```python
from build123d import *

# Parameters (mm, degrees)
CROQUIS1_W              = 30
CROQUIS1_H              = 35
CROQUIS1_R              = 1.5
CROQUIS1_R_2            = 2
SALIENTE_EXTRUIR1_DEPTH = 20
CROQUIS2_W              = 10
CROQUIS2_H              = 4
CORTAR_EXTRUIR1_DEPTH   = 41
CORTAR_EXTRUIR2_DEPTH   = 2
CORTAR_EXTRUIR3_DEPTH   = 3
CORTAR_EXTRUIR4_DEPTH   = 3
REDONDEO1_R             = 5
CROQUIS6_W              = 30
CROQUIS6_H              = 11
SALIENTE_EXTRUIR2_DEPTH = 10


with BuildPart() as part:
    # Croquis1 → Saliente-Extruir1 (new body)
    with BuildSketch(Plane(origin=(0, 0, 0), x_dir=(1, 0, 0), z_dir=(0, 1, 0))):
        with Locations((15, 17.5)):
            Rectangle(CROQUIS1_W, CROQUIS1_H)
        with Locations(Location((25, 30, 0), (0, 0, 270))):
            Circle(CROQUIS1_R, mode=Mode.SUBTRACT)
        with Locations(Location((5, 30, 0), (0, 0, 270))):
            Circle(CROQUIS1_R, mode=Mode.SUBTRACT)
        with Locations(Location((7.5, 5, 0), (0, 0, 270))):
            Circle(CROQUIS1_R_2, mode=Mode.SUBTRACT)
        with Locations(Location((22.5, 5, 0), (0, 0, 270))):
            Circle(CROQUIS1_R_2, mode=Mode.SUBTRACT)
    extrude(amount=SALIENTE_EXTRUIR1_DEPTH)

    # Croquis2 → Cortar-Extruir1 (cut)
    with BuildSketch(Plane(origin=(30, 0, 0), x_dir=(0, 0, -1), z_dir=(1, 0, 0))):
        with Locations((30, 13)):
            Rectangle(CROQUIS2_W, CROQUIS2_H)
    extrude(amount=-CORTAR_EXTRUIR1_DEPTH, mode=Mode.SUBTRACT)

    # Croquis3 → Cortar-Extruir2 (cut)
    with BuildSketch(Plane.XZ):
        Polygon((5, -33.117691454), (7.7, -31.558845727), (7.7, -28.441154273), (5, -26.882308546), (2.3, -28.441154273), (2.3, -31.558845727), align=None)
        Polygon((25, -33.117691454), (27.7, -31.558845727), (27.7, -28.441154273), (25, -26.882308546), (22.3, -28.441154273), (22.3, -31.558845727), align=None)
    extrude(amount=-CORTAR_EXTRUIR2_DEPTH, mode=Mode.SUBTRACT)

    # Croquis4 → Cortar-Extruir3 (cut)
    with BuildSketch(Plane.XZ):
        Polygon((7.5, -8.983716857), (10.95, -6.991858429), (10.95, -3.008141571), (7.5, -1.016283143), (4.05, -3.008141571), (4.05, -6.991858429), align=None)
        Polygon((22.5, -8.983716857), (25.95, -6.991858429), (25.95, -3.008141571), (22.5, -1.016283143), (19.05, -3.008141571), (19.05, -6.991858429), align=None)
    extrude(amount=-CORTAR_EXTRUIR3_DEPTH, mode=Mode.SUBTRACT)

    # Croquis5 → Cortar-Extruir4 (cut)
    with BuildSketch(Plane(origin=(0, 20, 0), x_dir=(1, 0, 0), z_dir=(0, 1, 0))):
        Polygon((22.5, 1.016283143), (19.05, 3.008141571), (19.05, 6.991858429), (22.5, 8.983716857), (25.95, 6.991858429), (25.95, 3.008141571), align=None)
        Polygon((4.05, 6.991858429), (7.5, 8.983716857), (10.95, 6.991858429), (10.95, 3.008141571), (7.5, 1.016283143), (4.05, 3.008141571), align=None)
    extrude(amount=-CORTAR_EXTRUIR4_DEPTH, mode=Mode.SUBTRACT)

    # Redondeo1
    redondeo1_edges = [part.edges().sort_by_distance(p)[0] for p in [
        (30, 10, 0),
        (0, 10, 0),
    ]]
    fillet(redondeo1_edges, radius=REDONDEO1_R)

    # Croquis6 → Saliente-Extruir2 (add)
    with BuildSketch(Plane(origin=(0, 0, -35), x_dir=(-1, 0, 0), z_dir=(0, 0, -1))):
        with Locations((-15, 5.5)):
            Rectangle(CROQUIS6_W, CROQUIS6_H)
    extrude(amount=SALIENTE_EXTRUIR2_DEPTH)


solid = part.part
```
Verification items for the finished model (mm, model axes). A direction names the side the tool comes from. Give positions to 0.01 mm unless a question says otherwise; leave off trailing zeros. Order: outer loops, then holes, each group sorted by start corner. A loop starts at its lowest first (then second) coordinate and runs counter-clockwise, first axis right, second up. Notation, with made-up numbers: (10.5, -34.75) -> (15.5, -34.75) arc R23 ccw to (15.5, -10.75) -> close; hole circle Ø7 at (61.5, -7). An arc over 180 degrees is marked (long way). One line per item, written item: value.
(1) Scan lines: line 1 along X through (y, z) = (8.5, -30); line 2 along Z through (x, y) = (7.5, 13); line 3 along Y through (x, z) = (27.5, -26.5). Record each from-to range of solid material in increasing order. Write a range as [from, to].
Final values:
line 1: [0, 3.5], [6.5, 23.5], [26.5, 30]
line 2: [-25, -7], [-3, 0]
line 3: [0, 11], [15, 20]
(2) Sectioned sample at D-D on x = 20. Record the cut outline in (y, z), then the cut area to 3 significant figures.
Final values:
outline: (0, -45) -> (11, -45) -> (11, -25) -> (15, -25) -> (15, -35) -> (20, -35) -> (20, -7.54) -> (17, -7.54) -> (17, -2.46) -> (20, -2.46) -> (20, 0) -> (0, 0) -> (0, -2.46) -> (3, -2.46) -> (3, -7.54) -> (0, -7.54) -> close
area: 740 mm^2
(3) Tool access check on faces 5 (the face through (9.2, 18.5, -8)), 6 (the face through (20.8, 1.5, -8)), 7 (the face through (15, 11, -35)). Record the directions out of +Z, -Z, +X, -X, +Y, -Y that give a thin tool (end or side, any length) a straight path to the whole face; none if there is none.
Final values:
face 5: +Y
face 6: -Y
face 7: -Z, +X, -X
(4) Draft check along Z on faces 1 (the face through (15, 6, -45)), 2 (the face through (9.2, 1.5, -8)), 3 (the face through (22.3, 1, -30)), 4 (the face through (0, 10, -25)). Enter one of: pulls with the +Z half, pulls with the -Z half, needs draft (parallel to the pull), parting line crosses it, or undercut.
Final values:
face 1: pulls with the -Z half
face 2: undercut
face 3: undercut
face 4: needs draft
(5) Sectioned sample at B-B on x = 14. Record the cut outline in (y, z).
Final values:
outline: (0, -45) -> (11, -45) -> (11, -25) -> (15, -25) -> (15, -35) -> (20, -35) -> (20, 0) -> (0, 0) -> close
(6) Sectioned sample at A-A on z = -30. Count the separate pieces of the cut face and the enclosed holes in it, then the cut area to 3 significant figures.
Final values:
separate pieces: 6
enclosed holes: 0
area: 374 mm^2
(7) Gauge pin test, flat end, axial feed: pin 1 (8 mm diameter, centred on x = 25.5, y = 16.5, fed in from -Z). Record the tip position at first contact, or that the pin passes through.
Final values:
pin 1: z = -35
(8) Sectioned sample at C-C on z = -42. Record the cut outline in (x, y).
Final values:
outline: (0, 0) -> (30, 0) -> (30, 11) -> (0, 11) -> close
